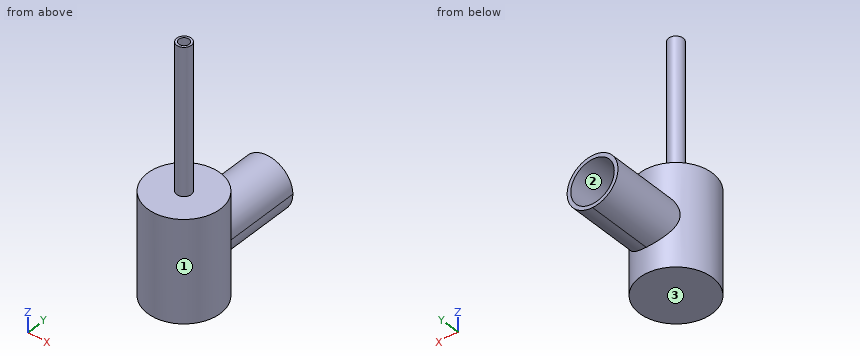
```python
from build123d import *

# Parameters (mm, degrees)
F0_R      = 63.5
F1_DEPTH  = 177.8
F3_DEPTH  = 177.8
F5_R      = 12.7
F6_DEPTH  = 254
F7_R      = 38.0000038218
F8_DEPTH  = 203.2
F9_R      = 9.036335061
F10_DEPTH = 228.6


with BuildPart() as f1:
    # F0 (on Top) → F1 (new body)
    with BuildSketch(Plane.XY):
        Circle(F0_R)
    extrude(amount=F1_DEPTH)

    # F2 (on Front) → F3 (join)
    with BuildSketch(Plane.XZ):
        with BuildLine():
            ThreePointArc((0, 44.45), (31.4308964237, 57.4691035763), (44.45, 88.9))
            ThreePointArc((44.45, 88.9), (-31.4308964237, 120.3308964237), (0, 44.45))
        make_face()
    extrude(amount=-F3_DEPTH)

    # F5 (on face) → F6 (join)
    with BuildSketch(Plane.XY.offset(177.8)):
        Circle(F5_R)
    extrude(amount=F6_DEPTH)

    # F7 (on face) → F8 (cut)
    with BuildSketch(Plane(origin=(0, 177.8, 0), x_dir=(-1, 0, 0), z_dir=(0, 1, 0))):
        with Locations((0, 88.7276828289)):
            Circle(F7_R)
    extrude(amount=-F8_DEPTH, mode=Mode.SUBTRACT)

    # F9 (on face) → F10 (cut)
    with BuildSketch(Plane.XY.offset(431.8)):
        Circle(F9_R)
    extrude(amount=-F10_DEPTH, mode=Mode.SUBTRACT)


solid = f1.part
```
Model file for the job. Use its own axes, mm. Face numbers are marked on the shaded views. Coordinates: 2 decimals unless noted, no trailing zeros. Loops run counter-clockwise (first coordinate to the right, second up) from the corner with the lowest first, then second, coordinate; pieces in that order, holes last. Notation, with made-up numbers: (-7, 39.25) - (11, 39.25) arc R19 ccw to (11, 44.25) - close; hole circle Ø6 at (21, -21.75). An arc over 180 degrees is marked (long way). Write item = value, one per line. Start each with the question number.
Item 1: Drop flat-ended pins along their axis: pin 1 Ø12 at (y, z) = (47.5, 140.5) entering from -X; pin 2 Ø10 at (y, z) = (-12, 62.5) entering from -X; pin 3 Ø3 at (y, z) = (132.5, 99.5) entering from +X. Give the stop position or say it passes through.
Item 2: Pull direction X, two halves, no side cores. Call the marked faces 1, 2 and 3: +X half, -X half, draft (parallel to the pull), parting line (faces both ways), or undercut.
Item 3: Saw through at C-C, the plane z = 38. List the corners of the cut face in (x, y).
Item 4: Saw through at A-A, the plane y = 20.5. List the corners of the cut face in (x, z).
Item 5: Saw through at D-D, the plane z = 190.5. List the corners of the cut face in (x, y), then the cut area to 3 significant figures.
Item 6: Wall check: probe 1 along Y at (x, z) = (-0.5, 411.5); probe 2 along Z at (x, y) = (2.5, 40); probe 3 along Z at (x, y) = (0, 79.5). Give the ranges that are in metal, low to high. Write a range as [from, to].
Item 7: Saw through at B-B, the plane x = 29.5. List the corners of the cut face in (y, z).
Answers:
q1.pin_1 = -48.06
q1.pin_2 = -63.11
q1.pin_3 = 43.51
q2.face_1 = parting line
q2.face_2 = undercut
q2.face_3 = draft
q3.outline = circle Ø127 at (0, 0)
q4.outline = (-60.1, 0) - (60.1, 0) - (60.1, 177.8) - (-60.1, 177.8) - close; hole circle Ø76 at (0, 88.73)
q5.outline = circle Ø25.4 at (0, 0)
q5.area = 507 mm2
q6.probe_1 = [-12.69, -9.02], [9.02, 12.69]
q6.probe_2 = [0, 50.81], [126.65, 177.8]
q6.probe_3 = [44.45, 50.73], [126.73, 133.35]
q7.outline = (-56.23, 0) - (56.23, 0) - (56.23, 55.65) - (177.8, 55.65) - (177.8, 64.77) - (-25.4, 64.77) - (-25.4, 112.68) - (177.8, 112.68) - (177.8, 122.15) - (56.23, 122.15) - (56.23, 177.8) - (-56.23, 177.8) - close
